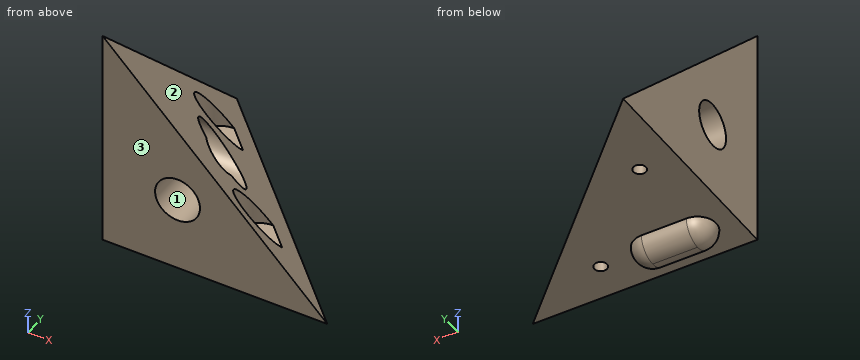
from build123d import *

# Parameters (mm, degrees)
CROQUIS1_W              = 30
CROQUIS1_H              = 30
CROQUIS1_R              = 0.85
SALIENTE_EXTRUIR1_DEPTH = 30
CHAFL_N1_START          = 17.320508076
CHAFL_N1_OUTLINE_W      = 52
CHAFL_N1_OUTLINE_H      = 46
CHAFL_N1_DEPTH          = 35.679491924
CORTAR_EXTRUIR1_REACH   = 51.759
CROQUIS2_R              = 3
CORTAR_EXTRUIR2_REACH   = 53.962
CROQUIS3_R              = 3
SALIENTE_EXTRUIR2_DEPTH = 2.5
REDONDEO1_R             = 2.5
CORTAR_EXTRUIR3_REACH   = 53.962
CROQUIS5_R              = 3


with BuildPart() as part:
    # Croquis1 → Saliente-Extruir1 (new body)
    with BuildSketch(Plane.XY):
        with Locations((15, 15)):
            Rectangle(CROQUIS1_W, CROQUIS1_H)
        with Locations((5, 17.928932188)):
            Circle(CROQUIS1_R, mode=Mode.SUBTRACT)
        with Locations((17.928932188, 5)):
            Circle(CROQUIS1_R, mode=Mode.SUBTRACT)
    extrude(amount=SALIENTE_EXTRUIR1_DEPTH)

    # Chaflán1: read off the stored shape, not the designer's step
    # Chaflán1 outline → Chaflán1 (cut)
    with BuildSketch(Plane(origin=(0, 0, 0), x_dir=(0.8164965809277258, -0.4082482904638636, -0.40824829046386285), z_dir=(0.5773502691896261, 0.5773502691896261, 0.5773502691896251)).offset(CHAFL_N1_START)):
        Rectangle(CHAFL_N1_OUTLINE_W, CHAFL_N1_OUTLINE_H)
    extrude(amount=CHAFL_N1_DEPTH, mode=Mode.SUBTRACT)

    # Croquis2 → Cortar-Extruir1 (cut, up to next)
    with BuildSketch(Plane(origin=(0, 0, 4), x_dir=(-1, 0, 0), z_dir=(0, 0, -1)), mode=Mode.PRIVATE) as cortar_extruir1_sk1:
        with Locations((-5, 17.928932188)):
            Circle(CROQUIS2_R)
    cortar_extruir1_tool1 = extrude(cortar_extruir1_sk1.sketch, amount=-CORTAR_EXTRUIR1_REACH, mode=Mode.PRIVATE) & part.part
    # Croquis2 → Cortar-Extruir1 (cut, up to next)
    with BuildSketch(Plane(origin=(0, 0, 4), x_dir=(-1, 0, 0), z_dir=(0, 0, -1)), mode=Mode.PRIVATE) as cortar_extruir1_sk2:
        with Locations((-17.928932188, 5)):
            Circle(CROQUIS2_R)
    cortar_extruir1_tool2 = extrude(cortar_extruir1_sk2.sketch, amount=-CORTAR_EXTRUIR1_REACH, mode=Mode.PRIVATE) & part.part
    add(cortar_extruir1_tool1.solids().sort_by_distance((5, 17.928932, 4))[0], mode=Mode.SUBTRACT)
    add(cortar_extruir1_tool2.solids().sort_by_distance((17.928932, 5, 4))[0], mode=Mode.SUBTRACT)

    # Cortar-Extruir2: up to this plane
    cortar_extruir2_end = Plane(origin=(0, 0, 30), z_dir=(0.5773502691896264, 0.5773502691896264, 0.5773502691896246))
    # Croquis3 → Cortar-Extruir2 (cut, up to the surface)
    with BuildSketch(Plane.ZY, mode=Mode.PRIVATE) as cortar_extruir2_sk1:
        with Locations((10, 10)):
            Circle(CROQUIS3_R)
    cortar_extruir2_tool1 = split(extrude(cortar_extruir2_sk1.sketch, amount=-CORTAR_EXTRUIR2_REACH, mode=Mode.PRIVATE), bisect_by=cortar_extruir2_end, keep=Keep.BOTH, mode=Mode.PRIVATE)
    add(cortar_extruir2_tool1.solids().sort_by_distance((0, 10, 10))[0], mode=Mode.SUBTRACT)

    # Croquis4 → Saliente-Extruir2 (add)
    with BuildSketch(Plane(origin=(0, 0, 0), x_dir=(-1, 0, 0), z_dir=(0, 0, -1))):
        with BuildLine():
            Line((-11, 7.5), (-5, 7.5))
            ThreePointArc((-5, 7.5), (-2.5, 5), (-5, 2.5))
            Line((-5, 2.5), (-11, 2.5))
            ThreePointArc((-11, 2.5), (-13.5, 5), (-11, 7.5))
        make_face()
    extrude(amount=SALIENTE_EXTRUIR2_DEPTH)

    # Redondeo1
    redondeo1_edges = [part.edges().sort_by_distance(p)[0] for p in [
        (8, 7.5, -2.5),
        (2.5, 5, -2.5),
        (8, 2.5, -2.5),
        (13.5, 5, -2.5),
    ]]
    fillet(redondeo1_edges, radius=REDONDEO1_R - 0.0001)  # a hair under: the kernel refuses the full size

    # Croquis5 → Cortar-Extruir3 (cut, up to next)
    with BuildSketch(Plane.XZ, mode=Mode.PRIVATE) as cortar_extruir3_sk1:
        with Locations(Location((10, 10, 0), (0, 0, 270))):
            Circle(CROQUIS5_R)
    cortar_extruir3_tool1 = extrude(cortar_extruir3_sk1.sketch, amount=-CORTAR_EXTRUIR3_REACH, mode=Mode.PRIVATE) & part.part
    add(cortar_extruir3_tool1.solids().sort_by_distance((10, 0, 10))[0], mode=Mode.SUBTRACT)


solid = part.part
Model file for the job. Use its own axes, mm. Face numbers are marked on the shaded views. Give positions to 0.01 mm unless a question says otherwise; leave off trailing zeros. Order: outer loops, then holes, each group sorted by start corner. A loop starts at its lowest first (then second) coordinate and runs counter-clockwise, first axis right, second up. Notation, with made-up numbers: (89.5, 71.5) - (139.5, 71.5) arc R26 cw to (139.5, 94.5) - close; hole circle Ø1 at (16.25, 38). An arc over 180 degrees is marked (long way). One line per item, written item: value.
Item 1: Slice it at A-A (z = 10.5). List the corners of the cut face in (x, y).
Response values:
outline: (0, 0) - (7.04, 0) - (7.04, 7.04) - (0, 7.04) - close; (0, 12.96) - (6.54, 12.96) - (4.53, 14.97) arc R3 cw to (2.04, 17.46) - (0, 19.5) - close; (12.96, 0) - (19.5, 0) - (17.46, 2.04) arc R3 cw to (14.97, 4.53) - (12.96, 6.54) - close
Item 2: Wall check: line 1 (Z direction, x = 10, y = 6); line 2 (Y direction, x = 4, z = 10); line 3 (X direction, y = 5.5, z = 17.5). Give the ranges that are in metal, low to high.
Response values:
line 1: -2.29 to 7, 13 to 14
line 2: 0 to 7, 13 to 15.1
line 3: 0 to 7
Item 3: Pin check, flat tips, straight feed: pin 1 Ø7 at (x, y) = (5, 17.93) entering from -Z; pin 2 Ø8 at (y, z) = (11.5, 6.5) entering from -X; pin 3 Ø8 at (y, z) = (20, 6.5) entering from +X; pin 4 Ø1.4 at (x, y) = (5, 17.93) entering from -Z. Stop position of each tip, or through.
Response values:
pin 1: z = 0
pin 2: x = 0
pin 3: x = 9.16
pin 4: through
Item 4: Slice it at B-B (y = 11). List the corners of the cut face in (x, z).
Response values:
outline: (0, 0) - (19, 0) - (11.83, 7.17) - (0, 7.17) - close; (0, 12.83) - (6.17, 12.83) - (0, 19) - close
Item 5: Slice it at D-D (y = 26). List the corners of the cut face in (x, z), then the cut area to 3 significant figures.
Response values:
outline: (0, 0) - (4, 0) - (0, 4) - close
area: 8.00 mm2
Item 6: Two-plate mould, pull along X, no slides. Class the marked faces 1, 2 and 3: released by +X, released by -X, zero draft, split by the parting line, or undercut.
Response values:
face 1: undercut
face 2: released by +X
face 3: zero draft
